Build history of the part. All positions in model axes, mm. A direction names the side the tool comes from. Round coordinates to 2 decimals unless told otherwise and drop trailing zeros. Write each loop counter-clockwise with the first axis right and the second up, starting at its lowest first coordinate (ties: lowest second). Pieces come first, ordered by that corner, then holes.
1) Wall check: probe 1 along Z at (x, y) = (-36.5, 42); probe 2 along Y at (x, z) = (-38.45, -11.4); probe 3 along X at (y, z) = (1.1, 0). Give the ranges that are in metal, low to high.
2) Pull direction Z, two halves, no side cores. Call faces 1 (the flat face through (-24, 17, -13.4)), 2 (the flat face through (-46.55, 14, 11)), 3 (the flat face through (-18, 2.75, 0)), 4 (the flat face through (-24, 19, 10.65)): +Z half, -Z half, draft (parallel to the pull), parting line (faces both ways), or undercut.
3) Saw through at D-D (z = 11.75). Write the cut outline in (x, y), plus the area to 3 significant figures.
4) Saw through at C-C (z = 1.5). Write the cut outline in (x, y), plus the area to 3 significant figures.
5) Which spindle directions (+Z, -Z, +X, -X, +Y, -Y) get a long thin tool onto all of the face, cutting with end or side? Do faces 5 (the flat face through (-24, 19, -10.65)), 6 (the flat face through (-18, 0, 0)), 7 (the flat face through (-42, 1, -4.25)). Say none if no direction does.
6) Saw through at A-A (y = 11). Write the cut outline in (x, z), plus the area to 3 significant figures.
7) Flat gauge pins, fed straight in: pin 1 (10.5 mm diameter, centred on x = -20, z = -3.5, fed in from +Y); pin 2 (6 mm diameter, centred on x = -4, z = -3, fed in from -Y). Where does each tip first touch, or does it go through?
8) Saw through at B-B (x = -2). Write the cut outline in (y, z).
from build123d import *

# Parameters (mm, degrees)
SKETCH1_R           = 4.25
BOSS_EXTRUDE1_DEPTH = 2.75
BOSS_EXTRUDE2_START = 13.4
SKETCH2_R           = 3.1
BOSS_EXTRUDE2_DEPTH = 2.75
BOSS_EXTRUDE3_START = -10.65
SKETCH2_2_R         = 3.1
BOSS_EXTRUDE3_DEPTH = 2.75


with BuildPart() as part:
    # Sketch1 → Boss-Extrude1 (new body)
    with BuildSketch(Plane(origin=(0, 0, 0), x_dir=(1, 0, 0), z_dir=(0, 1, 0))):
        with BuildLine():
            Line((-46.55, 4.25), (-36.5, 4.25))
            ThreePointArc((-36.5, 4.25), (-33.49479618, 3.00520382), (-32.25, 0))
            ThreePointArc((-32.25, 0), (-33.49479618, -3.00520382), (-36.5, -4.25))
            Line((-36.5, -4.25), (-46.55, -4.25))
            Line((-46.55, -4.25), (-46.55, -13.4))
            Line((-46.55, -13.4), (11.45, -13.4))
            Line((11.45, -13.4), (11.45, 13.4))
            Line((11.45, 13.4), (-46.55, 13.4))
            Line((-46.55, 13.4), (-46.55, 4.25))
        make_face()
        with Locations(Location((0, 0, 0), (0, 0, 270))):
            Circle(SKETCH1_R, mode=Mode.SUBTRACT)
    extrude(amount=BOSS_EXTRUDE1_DEPTH)

    # Sketch2 → Boss-Extrude2 (add)
    with BuildSketch(Plane.XY.offset(BOSS_EXTRUDE2_START)):
        with BuildLine():
            Line((-46.55, 0), (-46.55, 36.7))
            ThreePointArc((-46.55, 36.7), (-42.389803721, 43.777283846), (-34.182605767, 43.584718328))
            Line((-34.182605767, 43.584718328), (11.45, 15.3))
            Line((11.45, 15.3), (11.45, 0))
            Line((11.45, 0), (-46.55, 0))
        make_face()
        with Locations(Location((-38.45, 36.7, 0), (0, 0, 180))):
            Circle(SKETCH2_R, mode=Mode.SUBTRACT)
    extrude(amount=-BOSS_EXTRUDE2_DEPTH)

    # Sketch2<2> → Boss-Extrude3 (add)
    with BuildSketch(Plane.XY.offset(BOSS_EXTRUDE3_START)):
        with BuildLine():
            Line((-46.55, 0), (-46.55, 36.7))
            ThreePointArc((-46.55, 36.7), (-42.389803721, 43.777283846), (-34.182605767, 43.584718328))
            Line((-34.182605767, 43.584718328), (11.45, 15.3))
            Line((11.45, 15.3), (11.45, 0))
            Line((11.45, 0), (-46.55, 0))
        make_face()
        with Locations(Location((-38.45, 36.7, 0), (0, 0, 180))):
            Circle(SKETCH2_2_R, mode=Mode.SUBTRACT)
    extrude(amount=-BOSS_EXTRUDE3_DEPTH)


solid = part.part
Evaluation:
1. probe 1: z = -13.4 to -10.65, 10.65 to 13.4
1. probe 2: y = 0 to 33.6, 39.8 to 44.8
1. probe 3: x = -32.25 to -4.25, 4.25 to 11.45
2. face 1: -Z half
2. face 2: draft
2. face 3: undercut
2. face 4: undercut
3. outline: (-46.55, 0) - (11.45, 0) - (11.45, 15.3) - (-34.18, 43.58) arc R8.1 ccw to (-46.55, 36.7) - close; hole circle Ø6.2 at (-38.45, 36.7)
3. area: 1,850 mm2
4. outline: (-32.52, 0) - (-3.98, 0) - (-3.98, 2.75) - (-32.52, 2.75) - close; (3.98, 0) - (11.45, 0) - (11.45, 2.75) - (3.98, 2.75) - close
4. area: 99.1 mm2
5. face 5: +X, -X, +Y
5. face 6: +Z, -Z, +X, -X, -Y
5. face 7: -X, +Y, -Y
6. outline: (-46.55, -13.4) - (11.45, -13.4) - (11.45, -10.65) - (-46.55, -10.65) - close; (-46.55, 10.65) - (11.45, 10.65) - (11.45, 13.4) - (-46.55, 13.4) - close
6. area: 319 mm2
7. pin 1: stops at y = 2.75
7. pin 2: stops at y = 0
8. outline: (0, -13.4) - (23.64, -13.4) - (23.64, -10.65) - (2.75, -10.65) - (2.75, -3.75) - (0, -3.75) - close; (0, 3.75) - (2.75, 3.75) - (2.75, 10.65) - (23.64, 10.65) - (23.64, 13.4) - (0, 13.4) - close
